```python
from build123d import *

# Parameters (mm, degrees)
CHANNEL_START              = 63.5
SKETCH1_W                  = 12
SKETCH1_H                  = 12
CHANNEL_DEPTH              = 40
LIGHT_PATH_10MM_DEPTH      = 106.585273594
LIGHT_PATH_10MM_DEPTH_BACK = 106.585273594
SKETCH2_W                  = 10
SKETCH2_H                  = 10


with BuildPart() as part:
    # Sketch1 → Channel (new body)
    with BuildSketch(Plane(origin=(0, 0, 0), x_dir=(1, 0, 0), z_dir=(0, 1, 0)).offset(CHANNEL_START)):
        with Locations((14, 0)):
            Rectangle(SKETCH1_W, SKETCH1_H)
    extrude(amount=CHANNEL_DEPTH)

    # Sketch2 → Light_Path_10mm (cut, two sides: drawn at the far end of the back side and taken through both)
    with BuildSketch(Plane(origin=(0, 0, 0), x_dir=(1, 0, 0), z_dir=(0, 1, 0)).offset(-LIGHT_PATH_10MM_DEPTH_BACK)):
        with Locations((14, 0)):
            Rectangle(SKETCH2_W, SKETCH2_H)
    extrude(amount=LIGHT_PATH_10MM_DEPTH + LIGHT_PATH_10MM_DEPTH_BACK, mode=Mode.SUBTRACT)


solid = part.part
```
Here's how the part is built. I have some questions about the finished solid (model axes, mm). A direction names the side the tool comes from. Give positions to 0.01 mm unless a question says otherwise; leave off trailing zeros. Loops run counter-clockwise (first coordinate to the right, second up) from the corner with the lowest first, then second, coordinate; pieces in that order, holes last. Notation, with made-up numbers: M 68,61.25 L 124,61.25 A34 ccw 124,93.25 Z; hole C 12,27.5 d10. An arc over 180 degrees is marked long. Put each result on its own line as item: value. Start each with the question number.
(1) If we mould it in two halves opening along Z, with no side actions, what happens to faces 3 (the flat face through (14, 83, 6)), 4 (the flat face through (9, 83, 0)), 5 (the flat face through (8, 83, 0))? For each: +Z half, -Z half, draft (parallel to the pull), parting line (faces both ways), or undercut.
(2) I want a section at C-C on y = 67.5. Please give me the cut outline in (x, z).
(3) For faces 1 (the flat face through (8.6, 63.5, -0.1)), 2 (the flat face through (14, 83, 5)), which set-ups out of +Z, -Z, +X, -X, +Y, -Y let a thin tool reach every point of the face, with its end or its side?
(4) I want a section at B-B on z = -1.5. Please give me the cut outline in (x, y).
(5) I want a section at A-A on x = 16.5. Please give me the cut outline in (y, z).
(6) I need wall thicknesses on line 1 along X through (y, z) = (97, -1.5); line 2 along Z through (x, y) = (11.75, 77). Which ranges of each line are inside material? Lowest first, please. Write a range as [from, to].
Answer block:
1. face 3: +Z half
1. face 4: undercut
1. face 5: draft
2. outline: M 8,-6 L 20,-6 L 20,6 L 8,6 Z; hole M 9,-5 L 19,-5 L 19,5 L 9,5 Z
3. face 1: +Z, -Z, +X, -X, -Y
3. face 2: +Y, -Y
4. outline: M 8,63.5 L 9,63.5 L 9,103.5 L 8,103.5 Z; M 19,63.5 L 20,63.5 L 20,103.5 L 19,103.5 Z
5. outline: M 63.5,-6 L 103.5,-6 L 103.5,-5 L 63.5,-5 Z; M 63.5,5 L 103.5,5 L 103.5,6 L 63.5,6 Z
6. line 1: [8, 9], [19, 20]
6. line 2: [-6, -5], [5, 6]
